```python
from build123d import *

# Parameters (mm, degrees)
SKETCH_1_R          = 1.5
EXTRUDE_1_DEPTH     = 12
SKETCH_2_R          = 2.75
EXTRUDE_2_DEPTH     = 2.9
CUT_EXTRUDE_1_DEPTH = 1.5


with BuildPart() as part:
    # 草图1 → 凸台-拉伸1 (new body)
    with BuildSketch(Plane(origin=(0, 0, 0), x_dir=(1, 0, 0), z_dir=(0, 1, 0))):
        with Locations(Location((0, 0, 0), (0, 0, 270))):
            Circle(SKETCH_1_R)
    extrude(amount=EXTRUDE_1_DEPTH)

    # 草图2 → 凸台-拉伸2 (add)
    with BuildSketch(Plane.XZ):
        with Locations(Location((0, 0, 0), (0, 0, 270))):
            Circle(SKETCH_2_R)
    extrude(amount=EXTRUDE_2_DEPTH)

    # 草图3 → 切除-拉伸1 (cut)
    with BuildSketch(Plane.XZ.offset(2.9)):
        Polygon((1.25, 0.721687836), (0, 1.443375673), (-1.25, 0.721687836), (-1.25, -0.721687836), (0, -1.443375673), (1.25, -0.721687836), align=None)
    extrude(amount=-CUT_EXTRUDE_1_DEPTH, mode=Mode.SUBTRACT)


solid = part.part
```
For this review, take the finished solid that the model builds, in its own axes (mm). A direction names the side the tool comes from. Give positions to 0.01 mm unless a question says otherwise; leave off trailing zeros. Loops run counter-clockwise (first coordinate to the right, second up) from the corner with the lowest first, then second, coordinate; pieces in that order, holes last. Notation, with made-up numbers: M 83.25,21.5 L 136.25,21.5 A23 ccw 136.25,38.5 Z; hole C 65.25,-35 d2. An arc over 180 degrees is marked long. One line per item, written item: value. Start each with the question number.
Q1. Add section C-C (y = 10.75). Give the boundary of the cut face in (x, z), and give its area (3 significant figures).
Q2. Clearance check with flat-ended pins moving along their axes: pin 1 Ø1.2 at (x, z) = (0, 0) entering from -Y; pin 2 Ø1.5 at (y, z) = (3, 1) entering from +X; pin 3 Ø3 at (x, y) = (-1, 8) entering from +Z. State where each tip first meets the part, or that it passes through.
Q3. Machinability: for faces 4 (the face through (0, -1.4, 0)), 5 (the face through (-0.6, -2.9, 1.3)), 6 (the face through (-1.2, 0, -1.2)), which of the approach directions +Z, -Z, +X, -X, +Y, -Y give a long, thin tool a straight path to every point of the face, cutting with its end or side? Answer none if there is none.
Q4. For L1, parallel to Y at x = -1.7, z = 1.4; L2, parallel to Y at x = 1.15, z = 0.3; L3, parallel to X at y = 10.5, z = -0.05, list the stretches that pass through material, from the lowest coordinate up.
Q5. Add section B-B (x = -2.2). Give the boundary of the cut face in (y, z).
Q6. Draft analysis for pull direction Z (two halves, no side actions). For faces 1 (the face through (-0.63, -2.16, -1.08)), 2 (the face through (-2.685, -1.43, 0.596)), 3 (the face through (0, 12, 0)), state which applies: released by +Z, released by -Z, zero draft, split by the parting line, or undercut.
Q7. Add section A-A (z = 0). Give the boundary of the cut face in (x, y), and give its area (3 significant figures).
Q8. Add section D-D (x = 0.3). Give the boundary of the cut face in (y, z).
Reply:
1. outline: C 0,0 d3
1. area: 7.07 mm²
2. pin 1: y = -1.4
2. pin 2: x = 1.48
2. pin 3: z = 1.5
3. face 4: -Y
3. face 5: +Z, -Z, +X, -X, -Y
3. face 6: +Y
4. L1: -2.9 to 0
4. L2: -1.4 to 12
4. L3: -1.5 to 1.5
5. outline: M -2.9,-1.65 L 0,-1.65 L 0,1.65 L -2.9,1.65 Z
6. face 1: undercut
6. face 2: split by the parting line
6. face 3: zero draft
7. outline: M -2.75,-2.9 L -1.25,-2.9 L -1.25,-1.4 L 1.25,-1.4 L 1.25,-2.9 L 2.75,-2.9 L 2.75,0 L 1.5,0 L 1.5,12 L -1.5,12 L -1.5,0 L -2.75,0 Z
7. area: 48.2 mm²
8. outline: M -2.9,-2.73 L 0,-2.73 L 0,-1.47 L 12,-1.47 L 12,1.47 L 0,1.47 L 0,2.73 L -2.9,2.73 L -2.9,1.27 L -1.4,1.27 L -1.4,-1.27 L -2.9,-1.27 Z
